from build123d import *

# Parameters (mm, degrees)
F1_DEPTH = 30
F0_R     = 2.5
F0_R_2   = 1.375
F2_DEPTH = 4
F3_DEPTH = 8
F0_W     = 65
F0_H     = 36
F4_DEPTH = 2


with BuildPart() as f1:
    # F0 (on Top) → F1 (new body)
    with BuildSketch(Plane.XY):
        Polygon((31, 66), (31, 60), (35, 60), (35, 62), (33, 62), (33, 64), (35, 64), (35, 66), align=None)
    extrude(amount=F1_DEPTH)



with BuildPart() as f1b:
    # F0 (on Top) → F1, piece 2 (new body)
    with BuildSketch(Plane.XY):
        Polygon((50, 60), (54, 60), (54, 66), (50, 66), (50, 64), (52, 64), (52, 62), (50, 62), align=None)
    extrude(amount=F1_DEPTH)


with BuildPart() as f2:
    # F0 (on Top) → F2 (new body)
    with BuildSketch(Plane.XY):
        with Locations((3.5, 52.5)):
            Circle(F0_R)
        with Locations((3.5, 52.5)):
            Circle(F0_R_2, mode=Mode.SUBTRACT)
    extrude(amount=F2_DEPTH)

    # F0 (on Top) → F3 (join)
    with BuildSketch(Plane.XY):
        with Locations((3.5, 52.5)):
            Circle(F0_R_2)
    extrude(amount=F3_DEPTH)


with BuildPart() as f2b:
    # F0 (on Top) → F2, piece 2 (new body)
    with BuildSketch(Plane.XY):
        with Locations((61.5, 52.5)):
            Circle(F0_R)
        with Locations((61.5, 52.5)):
            Circle(F0_R_2, mode=Mode.SUBTRACT)
    extrude(amount=F2_DEPTH)

    # F0 (on Top) → F3, piece 2 (join)
    with BuildSketch(Plane.XY):
        with Locations((61.5, 52.5)):
            Circle(F0_R_2)
    extrude(amount=F3_DEPTH)


with BuildPart() as f2c:
    # F0 (on Top) → F2, piece 3 (new body)
    with BuildSketch(Plane.XY):
        with Locations((61.5, 3.5)):
            Circle(F0_R)
        with Locations((61.5, 3.5)):
            Circle(F0_R_2, mode=Mode.SUBTRACT)
    extrude(amount=F2_DEPTH)

    # F0 (on Top) → F3, piece 3 (join)
    with BuildSketch(Plane.XY):
        with Locations((61.5, 3.5)):
            Circle(F0_R_2)
    extrude(amount=F3_DEPTH)


with BuildPart() as f2d:
    # F0 (on Top) → F2, piece 4 (new body)
    with BuildSketch(Plane.XY):
        with Locations((3.5, 3.5)):
            Circle(F0_R)
        with Locations((3.5, 3.5)):
            Circle(F0_R_2, mode=Mode.SUBTRACT)
    extrude(amount=F2_DEPTH)

    # F0 (on Top) → F3, piece 4 (join)
    with BuildSketch(Plane.XY):
        with Locations((3.5, 3.5)):
            Circle(F0_R_2)
    extrude(amount=F3_DEPTH)


with BuildPart() as f1_1:
    add(f1.part)

    add(f1b.part)  # F4 merges F1b

    add(f2.part)  # F4 merges F2

    add(f2b.part)  # F4 merges F2b

    add(f2c.part)  # F4 merges F2c

    add(f2d.part)  # F4 merges F2d
    # F0 (on Top) → F4 (join)
    with BuildSketch(Plane.XY):
        Polygon((0, 28), (0, 0), (85, 0), (85, 28), (85, 56), (54, 56), (54, 60), (50, 60), (50, 62), (52, 62), (52, 64), (50, 64), (50, 66), (35, 66), (35, 64), (33, 64), (33, 62), (35, 62), (35, 60), (31, 60), (31, 56), (0, 56), align=None)
        with Locations((3.5, 3.5)):
            Circle(F0_R, mode=Mode.SUBTRACT)
        with Locations((61.5, 3.5)):
            Circle(F0_R, mode=Mode.SUBTRACT)
        with Locations((42.5, 28)):
            Rectangle(F0_W, F0_H, mode=Mode.SUBTRACT)
        with Locations((3.5, 52.5)):
            Circle(F0_R, mode=Mode.SUBTRACT)
        with Locations((61.5, 52.5)):
            Circle(F0_R, mode=Mode.SUBTRACT)
    extrude(amount=F4_DEPTH)


solid = f1_1.part
Work out the finished part from the listing and answer in its coordinate system (mm). A direction names the side the tool comes from. Round coordinates to 2 decimals unless told otherwise and drop trailing zeros. Write each loop counter-clockwise with the first axis right and the second up, starting at its lowest first coordinate (ties: lowest second). Pieces come first, ordered by that corner, then holes. Notation, with made-up numbers: (30, 77) - (89, 77) arc R11 ccw to (89, 83) - close; hole circle Ø7 at (-38, 34.5). An arc over 180 degrees is marked (long way). Answer in a Markdown table with one row per item. Add a question column.
1. A cutting plane is placed at A-A, the plane z = 27.75. Determine the outline of the cut face in (x, y).
2. A cutting plane is placed at B-B, the plane x = 61.5. Determine the outline of the cut face in (y, z) (3 decimals).
3. A cutting plane is placed at D-D, the plane y = 3.5. Determine the outline of the cut face in (x, z) (3 decimals).
4. For faces 5 (the flat face through (42, 48, 2)), 6 (the flat face through (10, 28, 1)), 7 (the flat face through (3, 53, 8)), 8 (the flat face through (33, 60, 16)), 9 (the flat face through (50, 61, 16)), determine the directions among +Z, -Z, +X, -X, +Y, -Y from which every point of the face is accessible in a straight line to the end or side of a thin tool.
5. Find the intervals of material crossed by line 1 along X through (y, z) = (22.5, 1.75); line 2 along Z through (x, y) = (49.5, 49), in increasing order. Write a range as from..to.
6. The mould has two halves that part along X. Classify faces 1 (the cylindrical face through (4.77, 2.97, 5.97)), 2 (the cylindrical face through (2.96, 50.06, 2.99)), 3 (the flat face through (0, 28, 1)), 4 (the flat face through (61, 53, 8)): +X half, -X half, draft (parallel to the pull), parting line (faces both ways), or undercut.
7. Given pin 1 (6 mm diameter, centred on x = 13.5, z = 5.5, fed in from +Y); pin 2 (0.6 mm diameter, centred on y = 65, z = 17, fed in from -X); pin 3 (0.6 mm diameter, centred on y = 60.5, z = 20.5, fed in from +X); pin 4 (2.5 mm diameter, centred on x = 61, y = 51.5, fed in from +Z), each flat-ended and moving along its own axis, determine where each tip first touches the part or whether it passes through.
8. A cutting plane is placed at C-C, the plane y = 24. Determine the outline of the cut face in (x, z).
Worked out:
| question | item | result |
|---|---|---|
| 1 | outline | (31, 60) - (35, 60) - (35, 62) - (33, 62) - (33, 64) - (35, 64) - (35, 66) - (31, 66) - close; (50, 60) - (54, 60) - (54, 66) - (50, 66) - (50, 64) - (52, 64) - (52, 62) - (50, 62) - close |
| 2 | outline | (0, 0) - (10, 0) - (10, 2) - (6, 2) - (6, 4) - (4.875, 4) - (4.875, 8) - (2.125, 8) - (2.125, 4) - (1, 4) - (1, 2) - (0, 2) - close; (46, 0) - (56, 0) - (56, 2) - (55, 2) - (55, 4) - (53.875, 4) - (53.875, 8) - (51.125, 8) - (51.125, 4) - (50, 4) - (50, 2) - (46, 2) - close |
| 3 | outline | (0, 0) - (85, 0) - (85, 2) - (64, 2) - (64, 4) - (62.875, 4) - (62.875, 8) - (60.125, 8) - (60.125, 4) - (59, 4) - (59, 2) - (6, 2) - (6, 4) - (4.875, 4) - (4.875, 8) - (2.125, 8) - (2.125, 4) - (1, 4) - (1, 2) - (0, 2) - close |
| 4 | face 5 | +Z |
| 4 | face 6 | +Z, -Z |
| 4 | face 7 | +Z, +X, -X, +Y, -Y |
| 4 | face 8 | +Z, +X, -X, -Y |
| 4 | face 9 | +Z, +Y, -Y |
| 5 | line 1 | 0..10, 75..85 |
| 5 | line 2 | 0..2 |
| 6 | face 1 | undercut |
| 6 | face 2 | undercut |
| 6 | face 3 | -X half |
| 6 | face 4 | draft |
| 7 | pin 1 | through |
| 7 | pin 2 | x = 31 |
| 7 | pin 3 | x = 54 |
| 7 | pin 4 | z = 8 |
| 8 | outline | (0, 0) - (10, 0) - (10, 2) - (0, 2) - close; (75, 0) - (85, 0) - (85, 2) - (75, 2) - close |
